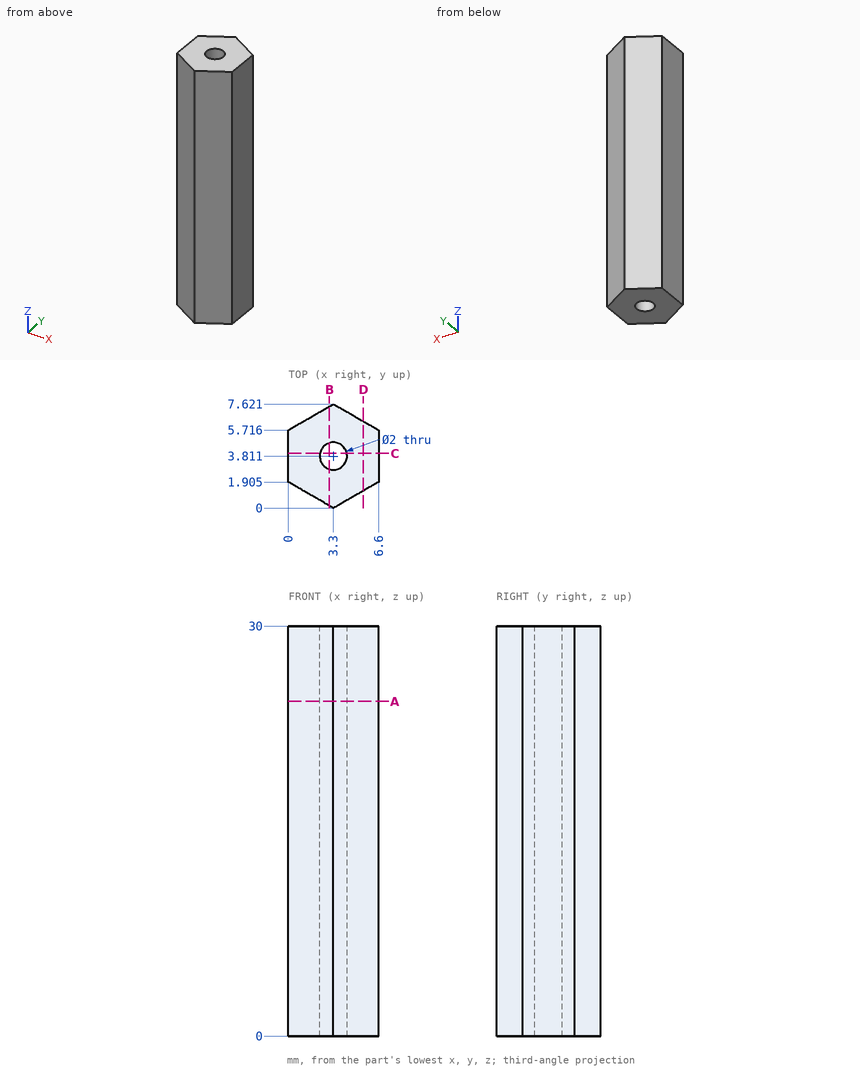
Geometry check sheet. Reference: drawing and pictorial views, mm from the part's lowest x, y, z. Round coordinates to 2 decimals unless told otherwise and drop trailing zeros. Order: outer loops, then holes, each group sorted by start corner. A loop starts at its lowest first (then second) coordinate and runs counter-clockwise, first axis right, second up. Notation, with made-up numbers: (48, -13.5) - (81, -13.5) arc R10 cw to (81, -7.5) - close; hole circle Ø10 at (2, 41.25). An arc over 180 degrees is marked (long way). Use a Markdown table: item, result. Add a question column.
1) Section check A-A (z = 24.5). Record the cut outline in (x, y) (1 decimal), then the cut area to 3 significant figures.
2) Section check C-C (y = 4). Record the cut outline in (x, z).
3) Thickness scan on line 1 along X through (y, z) = (4, 15.25); line 2 along Y through (x, z) = (3.5, 26.25) (1 decimal); line 3 along X through (y, z) = (5.75, 6.5) (1 decimal). Record the ranges inside material, lowest first.
4) Section check B-B (x = 3). Record the cut outline in (y, z) (1 decimal), then the cut area to 3 significant figures.
5) Section check D-D (x = 5.5). Record the cut outline in (y, z).
Established:
| question | item | result |
|---|---|---|
| 1 | outline | (0, 1.9) - (3.3, 0) - (6.6, 1.9) - (6.6, 5.7) - (3.3, 7.6) - (0, 5.7) - close; hole circle Ø2 at (3.3, 3.8) |
| 1 | area | 34.6 mm2 |
| 2 | outline | (0, 0) - (2.32, 0) - (2.32, 30) - (0, 30) - close; (4.28, 0) - (6.6, 0) - (6.6, 30) - (4.28, 30) - close |
| 3 | line 1 | 0 to 2.32, 4.28 to 6.6 |
| 3 | line 2 | 0.1 to 2.8, 4.8 to 7.5 |
| 3 | line 3 | 0.1 to 6.5 |
| 4 | outline | (0.2, 0) - (2.9, 0) - (2.9, 30) - (0.2, 30) - close; (4.8, 0) - (7.4, 0) - (7.4, 30) - (4.8, 30) - close |
| 4 | area | 161 mm2 |
| 5 | outline | (1.27, 0) - (6.35, 0) - (6.35, 30) - (1.27, 30) - close |
